Geometry: final body of the model. Coordinates: model frame, mm. A direction names the side the tool comes from. Coordinates: 2 decimals unless noted, no trailing zeros. Loops run counter-clockwise (first coordinate to the right, second up) from the corner with the lowest first, then second, coordinate; pieces in that order, holes last. Notation, with made-up numbers: M -7,23.25 L 35,23.25 A36 cw 35,57.25 Z; hole C 16,85 d6. An arc over 180 degrees is marked long. Write each question's results on one line, items separated by ' | '. Start each with the question number.
Autodesk Inventor part; units mm, degrees
ref_plane "YZ Plane" through (0, 0, 0) normal (1, 0, 0) x (0, 1, 0)
ref_plane "XZ Plane" through (0, 0, 0) normal (0, 1, 0) x (-1, 0, 0)
ref_plane "XY Plane" through (0, 0, 0) normal (0, 0, 1) x (1, 0, 0)
sketch "Sketch1" plane through (0, 0, 0) normal (0, 0, 1) x (1, 0, 0)
  arc A0 (-39.344, -1.4316) -> (39.344, -1.4316) centre (0, 0) ccw
  line L0 (-39.344, -1.4316) -> (-39.3671, -1.4316)
  line L1 (-39.344, -1.4316) -> (-52.044, -1.4316)
  line L2 (39.344, -1.4316) -> (52.044, -1.4316)
  arc A1 (-46.964, -22.4724) -> (46.964, -22.4724) centre (0, 0) ccw
  line L3 (-52.044, -1.4316) -> (-59.664, -1.4316)
  line L4 (52.044, -1.4316) -> (59.664, -1.4316)
  line L5 (39.344, -1.4316) -> (46.964, -1.4316)
  line L6 (46.964, -1.4316) -> (46.964, -22.4724)
  line L7 (-39.344, -1.4316) -> (-45.694, -1.4316)
  line L8 (-39.344, -1.4316) -> (-46.964, -1.4316)
  line L9 (-46.964, -1.4316) -> (-46.964, -22.4724)
  line L10 (-46.964, -7.7816) -> (-59.664, -7.7816)
  line L11 (-59.664, -7.7816) -> (-59.664, -1.4316)
  line L12 (46.964, -7.7816) -> (59.664, -7.7816)
  line L13 (59.664, -7.7816) -> (59.664, -1.4316)
  line L14 (46.964, -42.5386) -> (30.0181, -42.5386)
  line L15 (46.964, -22.4724) -> (46.964, -42.5386)
  line L16 (46.964, -42.5386) -> (-46.964, -42.5386)
  line L17 (-46.964, -42.5386) -> (-46.964, -22.4724)
  line L18 (-46.964, -42.5386) -> (46.964, -42.5386)
  line L19 (46.964, -42.5386) -> (46.964, -52.2316)
  line L20 (46.964, -52.2316) -> (-46.964, -52.2316)
  line L21 (-46.964, -52.2316) -> (-46.964, -42.5386)
  line L22 (-46.964, -22.4724) -> (-32.3263, -22.4724)
  line L23 (32.3263, -22.4724) -> (46.964, -22.4724)
  dimension "d0" = 78.74
  dimension "d1" = 12.7
  dimension "d2" = 12.7
  dimension "d4" = 7.62
  dimension "d5" = 7.62
  dimension "d6" = 7.62
  dimension "d7" = 7.62
  dimension "d8" = 6.35
  dimension "d9" = 6.35
  dimension "d20" = 50.8
extrude "Extrusion1" add sketch "Sketch1" along normal blind 12.7
sketch "Sketch2" plane through (-59.664, -1.4316, 0) normal (0, 1, 0) x (1, 0, 0)
  line L0 (20.32, 0) -> (0, 0)
  line L1 (0, 0) -> (20.32, 0)
  circle A0 centre (7.62, -6.35) radius 4.064
  circle A1 centre (111.7079, -6.35) radius 4.064
  line L2 (99.0079, 0) -> (99.0079, -12.7)
  line L3 (20.32, 0) -> (20.32, -12.7)
  point P0 (59.664, 0)
  dimension "d14" = 12.7
  dimension "d15" = 12.7
  dimension "d16" = 8.128
  dimension "d17" = 8.128
extrude "Extrusion2" cut sketch "Sketch2" against normal blind 25.4
sketch "Sketch3" plane through (0, 0, 12.7) normal (0, 0, 1) x (1, 0, 0)
  arc A0 (-39.344, -1.4316) -> (39.344, -1.4316) centre (0, 0) ccw
  arc A1 (39.344, -1.4316) -> (-39.344, -1.4316) centre (0, 0) ccw
  line L0 (-59.664, -7.7816) -> (-46.964, -7.7816)
  line L1 (46.964, -52.2316) -> (46.964, -7.7816)
  arc A2 (-46.964, -7.7816) -> (46.964, -7.7816) centre (0, 0) ccw
  line L2 (-46.964, -7.7816) -> (-46.964, -52.2316)
  line L3 (46.964, -7.7816) -> (-46.964, -7.7816)
  line L4 (-46.964, -7.7816) -> (-46.964, -52.2316)
  line L5 (-46.964, -52.2316) -> (46.964, -52.2316)
  line L6 (46.964, -52.2316) -> (46.964, -7.7816)
extrude "Extrusion3" cut sketch "Sketch3" against normal blind 25.4 contours A2 L1 L5 L2
properties part number "MOTOR MOUNT REAL TOP E3O MOTOR"
Item 1: Pull-direction query (X, two-part tool) for faces 1 (the cylindrical face through (-0.937, -47.595, 6.439)), 2 (the cylindrical face through (-48.168, -4.562, 5.129)), 3 (the flat face through (59.664, -5, 6)), 4 (the cylindrical face through (55.92, -4.56, 5.13)); classes: released by +X, released by -X, zero draft, split by the parting line, or undercut.
Item 2: Section C-C, the plane x = 52. Return loops of the section in (y, z).
Item 3: Set-up query: faces 5 (the cylindrical face through (0.85, -39.36, 6.26)), 6 (the flat face through (-56, -7.782, 8)), 7 (the flat face through (56, -7.782, 8)). Return all of +Z, -Z, +X, -X, +Y, -Y with unobstructed straight access to the full face (end or side cutting, diameter ignored); none if empty.
Item 4: Ray query, L1, parallel to X at y = -2.25, z = 6.35; L2, parallel to X at y = -4.75, z = 6.35; L3, parallel to X at y = -31, z = 8.5. Return the intervals inside material, ascending. Write a range as [from, to].
Item 5: Contact query for flat-ended pins moving along their axis: P1, Ø8, axis at x = -26, y = -21.5, coming from the -Z side; P2, Ø4, axis at x = -51.5, z = 3, coming from the -Y side; P3, Ø6, axis at x = -39.5, z = 11, coming from the -Y side; P4, Ø3, axis at y = -37.5, z = 4, coming from the -X side. Output: stop coordinate, or through.
Item 6: Section B-B, the plane y = -27. Return loops of the section in (x, z), plus the area to 3 significant figures.
Solutions:
1) face 1: split by the parting line | face 2: undercut | face 3: released by +X | face 4: undercut
2) outline: M -7.78,0 L -1.43,0 L -1.43,2.29 L -7.78,2.29 Z; M -7.78,10.41 L -1.43,10.41 L -1.43,12.7 L -7.78,12.7 Z
3) face 5: +Z, -Z, +Y | face 6: +Z, -Z, -X, -Y | face 7: +Z, -Z, +X, -Y
4) L1: x = [-59.66, -56.11], [-47.98, -39.31], [39.31, 47.98], [56.11, 59.66] | L2: x = [-59.66, -56.11], [-47.98, -39.08], [39.08, 47.98], [56.11, 59.66] | L3: x = [-36.13, -24.27], [24.27, 36.13]
5) P1: passes through | P2: stops at y = -7.78 | P3: stops at y = -30.56 | P4: stops at x = -31.15
6) outline: M -39.21,0 L -28.65,0 L -28.65,12.7 L -39.21,12.7 Z; M 28.65,0 L 39.21,0 L 39.21,12.7 L 28.65,12.7 Z | area: 268 mm²
